Could you check a few things on this drawing? It's one solid part, dimensions in mm from its lowest x, y, z. A direction names the side the tool comes from. Round coordinates to 2 decimals unless told otherwise and drop trailing zeros. Loops run counter-clockwise (first coordinate to the right, second up) from the corner with the lowest first, then second, coordinate; pieces in that order, holes last. Notation, with made-up numbers: M 48.25,-5 L 67.25,-5 A14 cw 67.25,22 Z; hole C 29.5,12.5 d11. An arc over 180 degrees is marked long. Answer as a JSON object with one key per item and string values.
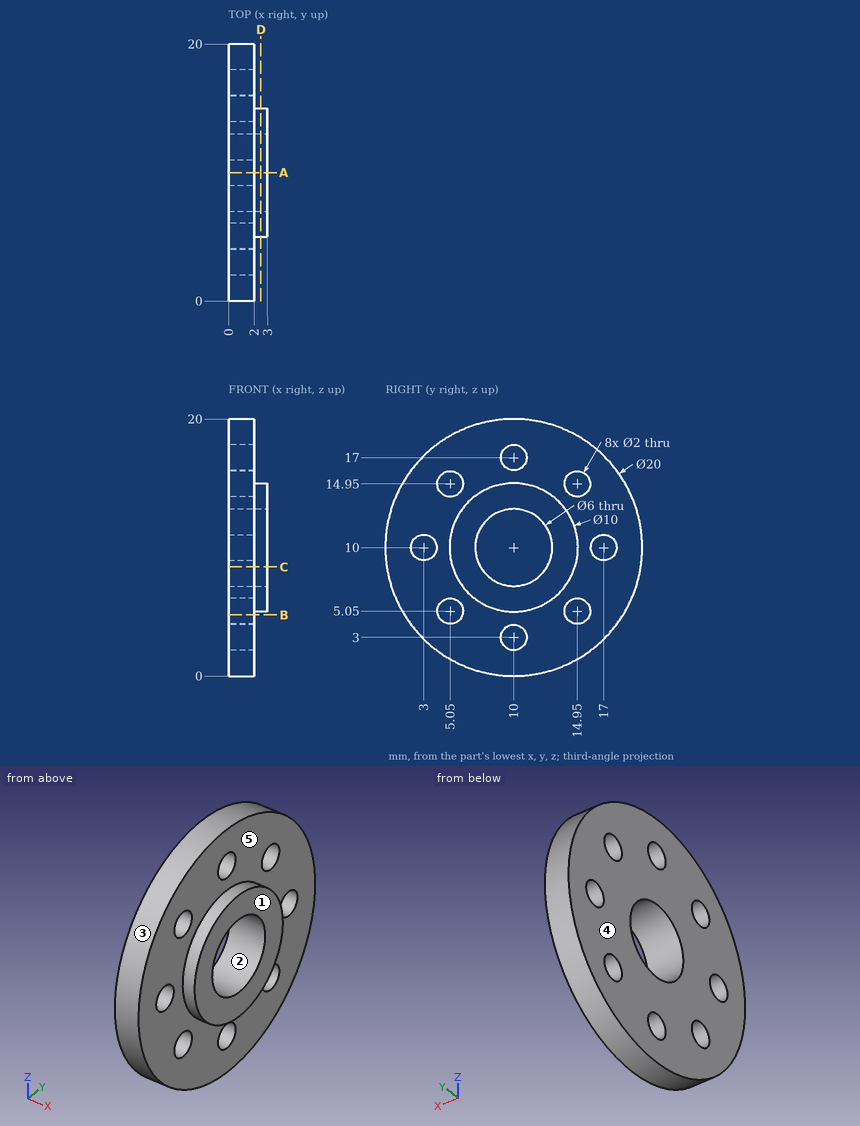
Item 1: I want a section at A-A, the plane y = 10. Please give me the cut outline in (x, z).
Resolved:
{"outline": "M 0,0 L 2,0 L 2,2 L 0,2 Z; M 0,4 L 2,4 L 2,5 L 3,5 L 3,7 L 0,7 Z; M 0,13 L 3,13 L 3,15 L 2,15 L 2,16 L 0,16 Z; M 0,18 L 2,18 L 2,20 L 0,20 Z"}
Item 2: Please list where these lines run through material, in increasing order: probe 1 along Y at (x, z) = (0.5, 10); probe 2 along Z at (x, y) = (1.25, 5.25); probe 3 along Y at (x, z) = (1, 15.5) (1 decimal). Write a range as from..to.
Resolved:
{"probe 1": "0..2, 4..7, 13..16, 18..20", "probe 2": "1.2..4.07, 6.03..13.97, 15.93..18.8", "probe 3": "1.6..4.2, 5.9..14.1, 15.8..18.4"}
Item 3: I'm going to push flat-ended pins straight in: pin 1 Ø2.5 at (y, z) = (5.05, 5.05) entering from +X; pin 2 Ø9.5 at (y, z) = (10, 10) entering from -X; pin 3 Ø1.5 at (x, z) = (2, 5.5) entering from -Y. Where does each tip first touch, or does it pass through?
Resolved:
{"pin 1": "x = 2", "pin 2": "x = 0", "pin 3": "y = 0.73"}
Item 4: If we mould it in two halves opening along Y, with no side actions, what happens to the marked faces 1, 2 and 3? For each: pulls with the +Y half, pulls with the -Y half, needs draft (parallel to the pull), parting line crosses it, or undercut.
Resolved:
{"face 1": "needs draft", "face 2": "undercut", "face 3": "parting line crosses it"}
Item 5: I want a section at B-B, the plane z = 4.75. Please give me the cut outline in (x, y).
Resolved:
{"outline": "M 0,1.49 L 2,1.49 L 2,4.1 L 0,4.1 Z; M 0,6 L 2,6 L 2,14 L 0,14 Z; M 0,15.9 L 2,15.9 L 2,18.51 L 0,18.51 Z"}
Item 6: On a 3-axis mill with a long thin cutter (end or side, diameter ignored), from which of +Z, -Z, +X, -X, +Y, -Y can I reach the whole of each face in a straight line? I mean the marked faces 4 and 5. Say none if no direction works.
Resolved:
{"face 4": "+Z, -Z, -X, +Y, -Y", "face 5": "+X"}
Item 7: I want a section at C-C, the plane z = 8.5. Please give me the cut outline in (x, y), then the cut area to 3 significant figures.
Resolved:
{"outline": "M 0,0.11 L 2,0.11 L 2,5.23 L 3,5.23 L 3,7.4 L 0,7.4 Z; M 0,12.6 L 3,12.6 L 3,14.77 L 2,14.77 L 2,19.89 L 0,19.89 Z", "area": "33.5 mm²"}
Item 8: I want a section at D-D, the plane x = 2.5. Please give me the cut outline in (y, z).
Resolved:
{"outline": "C 10,10 d10; hole C 10,10 d6"}
